Design review of the part built by this model. Coordinates are the model's own, in mm. Round coordinates to 2 decimals unless told otherwise and drop trailing zeros. Order: outer loops, then holes, each group sorted by start corner. A loop starts at its lowest first (then second) coordinate and runs counter-clockwise, first axis right, second up.
from build123d import *

# Parameters (mm, degrees)
F1_DEPTH = 9.525


with BuildPart() as f1:
    # F0 (on Top) → F1 (new body)
    with BuildSketch(Plane.XY):
        with BuildLine():
            Line((0, 152.4), (0, 0))
            Line((0, 0), (311.15, 0))
            Line((311.15, 0), (311.15, 25.4))
            Line((311.15, 25.4), (160.901719, 344.192777))
            ThreePointArc((160.901719, 344.192777), (162.712271, 338.912413), (163.325663, 333.364072))
            ThreePointArc((163.325663, 333.364072), (155.552888, 315.076345), (136.99173, 307.981248))
            ThreePointArc((136.99173, 307.981248), (136.059369, 307.981167), (135.137047, 308.117615))
            ThreePointArc((135.137047, 308.117615), (112.564078, 334.760493), (137.925663, 358.764072))
            Line((137.925663, 358.764072), (55.782063, 358.764072))
            ThreePointArc((55.782063, 358.764072), (73.742576, 351.324585), (81.182063, 333.364072))
            ThreePointArc((81.182063, 333.364072), (53.695638, 308.04991), (30.724833, 337.522821))
            Line((30.724833, 337.522821), (0, 152.4))
        make_face()
        with BuildLine():
            ThreePointArc((83.451245, 267.376207), (107.748281, 290.885778), (137.465097, 274.762605))
            Line((137.465097, 274.762605), (217.824916, 104.257293))
            ThreePointArc((217.824916, 104.257293), (219.861787, 98.316884), (220.551853, 92.075))
            ThreePointArc((220.551853, 92.075), (212.182429, 71.869424), (191.976853, 63.5))
            Line((191.976853, 63.5), (83.315653, 63.5))
            ThreePointArc((83.315653, 63.5), (61.487623, 73.641806), (55.150963, 96.861752))
            Line((55.150963, 96.861752), (83.410288, 267.129432))
            ThreePointArc((83.410288, 267.129432), (83.430497, 267.252864), (83.451245, 267.376207))
        make_face(mode=Mode.SUBTRACT)
        with BuildLine():
            ThreePointArc((55.782063, 358.764072), (39.357573, 352.739214), (30.724833, 337.522821))
            ThreePointArc((30.724833, 337.522821), (53.695638, 308.04991), (81.182063, 333.364072))
            ThreePointArc((81.182063, 333.364072), (73.742576, 351.324585), (55.782063, 358.764072))
        make_face()
        with BuildLine():
            ThreePointArc((163.325663, 333.364072), (162.712271, 338.912413), (160.901719, 344.192777))
            ThreePointArc((160.901719, 344.192777), (151.529172, 354.81412), (137.925663, 358.764072))
            ThreePointArc((137.925663, 358.764072), (112.564078, 334.760493), (135.137047, 308.117615))
            ThreePointArc((135.137047, 308.117615), (132.555806, 319.270684), (142.875, 314.314072))
            ThreePointArc((142.875, 314.314072), (141.177216, 309.992107), (136.99173, 307.981248))
            ThreePointArc((136.99173, 307.981248), (155.552888, 315.076345), (163.325663, 333.364072))
        make_face()
    extrude(amount=F1_DEPTH)


solid = f1.part
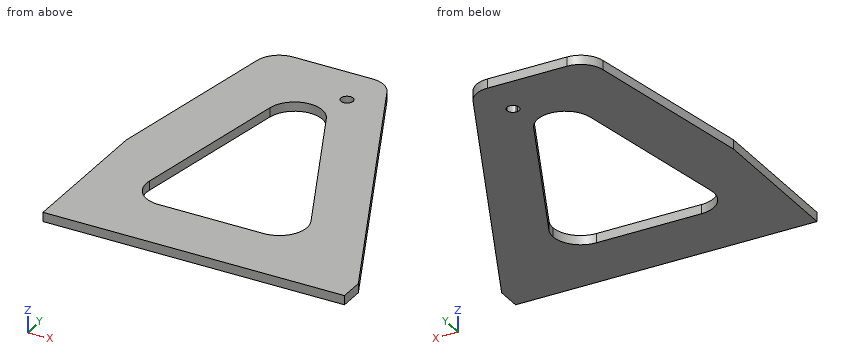
1) Take a section at B-B on x = 156.5. Give the boundary of the cut face in (y, z) (3 decimals), plus the area to 3 significant figures.
Results:
outline: (0, 0) - (63.5, 0) - (63.5, 9.525) - (0, 9.525) - close; (234.375, 0) - (350.689, 0) - (350.689, 9.525) - (234.375, 9.525) - close
area: 1,710 mm2
2) Take a section at D-D on x = 273. Give the boundary of the cut face in (y, z) (3 decimals), plus the area to 3 significant figures.
Results:
outline: (0, 0) - (106.346, 0) - (106.346, 9.525) - (0, 9.525) - close
area: 1,010 mm2
3) Take a section at C-C on y = 124.5. Give the boundary of the cut face in (x, z) (3 decimals).
Results:
outline: (0, 0) - (59.738, 0) - (59.738, 9.525) - (0, 9.525) - close; (208.284, 0) - (264.444, 0) - (264.444, 9.525) - (208.284, 9.525) - close
4) To check wall thickness, follow line 1 along X through (y, z) = (244, 3); line 2 along X through (y, z) = (279, 4); line 3 along Y through (x, z) = (185.5, 7.5). State the ranges of each line that lie inside material, in increasing order.
Results:
line 1: x = 15.2 to 79.57, 151.96 to 208.12
line 2: x = 21.01 to 88.24, 135 to 191.63
line 3: y = 0 to 63.5, 172.84 to 292
5) Take a section at A-A on z = 3. Give the boundary of the cut face in (x, y) (3 decimals), plus the area to 3 significant figures.
Results:
outline: (0, 0) - (311.15, 0) - (311.15, 25.4) - (160.902, 344.193) arc R25.4 ccw to (137.926, 358.764) - (55.782, 358.764) arc R25.4 ccw to (30.725, 337.523) - (0, 152.4) - close; hole (55.151, 96.862) arc R28.575 ccw to (83.316, 63.5) - (191.977, 63.5) arc R28.575 ccw to (220.552, 92.075) arc R28.575 ccw to (217.825, 104.257) - (137.465, 274.763) arc R28.575 ccw to (83.451, 267.376) arc R28.636 ccw to (83.41, 267.129) - close; hole (135.137, 308.118) arc R6.35 ccw to (136.992, 307.981) arc R6.35 ccw (long way) to start
area: 56,400 mm2
6) Clearance check with flat-ended pins moving along their axes: P1, Ø10, axis at x = 81.5, y = 214.5, coming from the -Z side; P2, Ø1, axis at y = 103.5, z = 2, coming from the +X side. State where each tip first meets the part, or that it passes through.
Results:
P1: passes through
P2: stops at x = 274.58
